from build123d import *

# Parameters (mm, degrees)
SKETCH_1_W          = 103.2
SKETCH_1_H          = 55.2
SKETCH_1_R          = 1.6
EXTRUDE_1_DEPTH     = 3
FILLET_1_R          = 2
SKETCH_2_W          = 10
SKETCH_2_H          = 8
EXTRUDE_2_DEPTH     = 10
SKETCH_3_W          = 10
SKETCH_3_H          = 7.8
SKETCH_3_W_2        = 7.907318886
SKETCH_3_H_2        = 12.798311125
SKETCH_3_W_3        = 8.73556964
SKETCH_3_H_3        = 16.298311125
SKETCH_3_H_4        = 8.73556964
EXTRUDE_3_DEPTH     = 3
SKETCH_4_R          = 2.5
SKETCH_4_W          = 7
SKETCH_4_H          = 14
SKETCH_4_W_2        = 5
SKETCH_4_H_2        = 12
EXTRUDE_4_DEPTH     = 8
SKETCH_5_R          = 0.25
EXTRUDE_5_DEPTH     = 7
SKETCH_6_R          = 5
EXTRUDE_6_DEPTH     = 12
SKETCH_7_W          = 36.530578683
SKETCH_7_H          = 32.729234011
CUT_EXTRUDE_1_DEPTH = 60.73541663


with BuildPart() as part:
    # 草图1 → 凸台-拉伸1 (new body)
    with BuildSketch(Plane(origin=(0, 0, 0), x_dir=(1, 0, 0), z_dir=(0, 1, 0))):
        Rectangle(SKETCH_1_W, SKETCH_1_H)
        with Locations(Location((-46.6, 21.6, 0), (0, 0, 270))):
            Circle(SKETCH_1_R, mode=Mode.SUBTRACT)
        with Locations(Location((46.6, 21.6, 0), (0, 0, 270))):
            Circle(SKETCH_1_R, mode=Mode.SUBTRACT)
        with Locations(Location((46.6, -21.6, 0), (0, 0, 270))):
            Circle(SKETCH_1_R, mode=Mode.SUBTRACT)
        with Locations(Location((-46.6, -21.6, 0), (0, 0, 270))):
            Circle(SKETCH_1_R, mode=Mode.SUBTRACT)
    extrude(amount=EXTRUDE_1_DEPTH)

    # 圆角1
    fillet_1_edges = [part.edges().sort_by_distance(p)[0] for p in [
        (51.6, 1.5, 27.6),
        (-51.6, 1.5, 27.6),
        (-51.6, 1.5, -27.6),
        (51.6, 1.5, -27.6),
    ]]
    fillet(fillet_1_edges, radius=FILLET_1_R)

    # 草图2 → 凸台-拉伸2 (add)
    with BuildSketch(Plane(origin=(0, 3, 0), x_dir=(1, 0, 0), z_dir=(0, 1, 0))):
        with Locations((-45.6, 13)):
            Rectangle(SKETCH_2_W, SKETCH_2_H)
        with Locations((45.6, 13)):
            Rectangle(SKETCH_2_W, SKETCH_2_H)
        with Locations((45.6, -13)):
            Rectangle(SKETCH_2_W, SKETCH_2_H)
        with Locations((-45.6, -13)):
            Rectangle(SKETCH_2_W, SKETCH_2_H)
    extrude(amount=EXTRUDE_2_DEPTH)

    # 草图3 → 凸台-拉伸3 (add)
    with BuildSketch(Plane(origin=(0, 3, 0), x_dir=(1, 0, 0), z_dir=(0, 1, 0))):
        with Locations((31, 21)):
            Rectangle(SKETCH_3_W, SKETCH_3_H)
        with Locations((-31, 21)):
            Rectangle(SKETCH_3_W, SKETCH_3_H)
        with Locations((31, 7)):
            Rectangle(SKETCH_3_W, SKETCH_3_H)
        with Locations((31, -7)):
            Rectangle(SKETCH_3_W, SKETCH_3_H)
        with Locations((31, -21)):
            Rectangle(SKETCH_3_W, SKETCH_3_H)
        with Locations((-31, 7)):
            Rectangle(SKETCH_3_W, SKETCH_3_H)
        with Locations((-31, -7)):
            Rectangle(SKETCH_3_W, SKETCH_3_H)
        with Locations((-31, -21)):
            Rectangle(SKETCH_3_W, SKETCH_3_H)
        with Locations((7.453659443, -2.077902605)):
            Rectangle(SKETCH_3_W_2, SKETCH_3_H_2)
        with Locations((-7.86778482, -3.827902605)):
            Rectangle(SKETCH_3_W_3, SKETCH_3_H_3)
        with Locations((-7.86778482, -20.98502184)):
            Rectangle(SKETCH_3_W_3, SKETCH_3_H_4)
    extrude(amount=EXTRUDE_3_DEPTH)

    # 草图4 → 凸台-拉伸4 (add)
    # profile 1 of 3: a face of its own
    with BuildSketch(Plane(origin=(0, 3, 0), x_dir=(1, 0, 0), z_dir=(0, 1, 0))):
        with Locations(Location((2, -24, 0), (0, 0, 90))):
            Circle(SKETCH_4_R)
    # profile 2 of 3: a face of its own
    with BuildSketch(Plane(origin=(0, 3, 0), x_dir=(1, 0, 0), z_dir=(0, 1, 0))):
        with Locations((-7, 17.9)):
            Rectangle(SKETCH_4_W, SKETCH_4_H)
        with Locations((-7, 17.9)):
            Rectangle(SKETCH_4_W_2, SKETCH_4_H_2, mode=Mode.SUBTRACT)
    # profile 3 of 3: a face of its own
    with BuildSketch(Plane(origin=(0, 3, 0), x_dir=(1, 0, 0), z_dir=(0, 1, 0))):
        with Locations((7, 17.9)):
            Rectangle(SKETCH_4_W, SKETCH_4_H)
        with Locations((7, 17.9)):
            Rectangle(SKETCH_4_W_2, SKETCH_4_H_2, mode=Mode.SUBTRACT)
    extrude(amount=EXTRUDE_4_DEPTH)

    # 草图5 → 凸台-拉伸5 (add)
    with BuildSketch(Plane(origin=(0, 3, 0), x_dir=(1, 0, 0), z_dir=(0, 1, 0))):
        with Locations(Location((-8.182313365, 22.9, 0), (0, 0, 90))):
            Circle(SKETCH_5_R)
        with Locations(Location((-5.817686635, 22.9, 0), (0, 0, 90))):
            Circle(SKETCH_5_R)
        with Locations(Location((-8.182313365, 20.4, 0), (0, 0, 90))):
            Circle(SKETCH_5_R)
        with Locations(Location((-5.817686635, 20.4, 0), (0, 0, 90))):
            Circle(SKETCH_5_R)
        with Locations(Location((-8.182313365, 17.9, 0), (0, 0, 90))):
            Circle(SKETCH_5_R)
        with Locations(Location((-5.817686635, 17.9, 0), (0, 0, 90))):
            Circle(SKETCH_5_R)
        with Locations(Location((-8.182313365, 15.4, 0), (0, 0, 90))):
            Circle(SKETCH_5_R)
        with Locations(Location((-5.817686635, 15.4, 0), (0, 0, 90))):
            Circle(SKETCH_5_R)
        with Locations(Location((-8.182313365, 12.9, 0), (0, 0, 90))):
            Circle(SKETCH_5_R)
        with Locations(Location((-5.817686635, 12.9, 0), (0, 0, 90))):
            Circle(SKETCH_5_R)
        with Locations(Location((5.817686635, 12.9, 0), (0, 0, 90))):
            Circle(SKETCH_5_R)
        with Locations(Location((8.182313365, 12.9, 0), (0, 0, 90))):
            Circle(SKETCH_5_R)
        with Locations(Location((5.817686635, 15.4, 0), (0, 0, 90))):
            Circle(SKETCH_5_R)
        with Locations(Location((8.182313365, 15.4, 0), (0, 0, 90))):
            Circle(SKETCH_5_R)
        with Locations(Location((5.817686635, 17.9, 0), (0, 0, 90))):
            Circle(SKETCH_5_R)
        with Locations(Location((8.182313365, 17.9, 0), (0, 0, 90))):
            Circle(SKETCH_5_R)
        with Locations(Location((5.817686635, 20.4, 0), (0, 0, 90))):
            Circle(SKETCH_5_R)
        with Locations(Location((8.182313365, 20.4, 0), (0, 0, 90))):
            Circle(SKETCH_5_R)
        with Locations(Location((8.182313365, 22.9, 0), (0, 0, 90))):
            Circle(SKETCH_5_R)
        with Locations(Location((5.817686635, 22.9, 0), (0, 0, 90))):
            Circle(SKETCH_5_R)
    extrude(amount=EXTRUDE_5_DEPTH)

    # 草图6 → 凸台-拉伸6 (add)
    with BuildSketch(Plane(origin=(0, 3, 0), x_dir=(1, 0, 0), z_dir=(0, 1, 0))):
        with Locations(Location((8.346758727, -16.964516113, 0), (0, 0, 90))):
            Circle(SKETCH_6_R)
    extrude(amount=EXTRUDE_6_DEPTH)

    # 草图7 → 切除-拉伸1 (cut, through all)
    with BuildSketch(Plane(origin=(0, 3, 0), x_dir=(1, 0, 0), z_dir=(0, 1, 0))):
        with Locations((40.691092522, -17.246006906)):
            Rectangle(SKETCH_7_W, SKETCH_7_H)
    extrude(amount=CUT_EXTRUDE_1_DEPTH, mode=Mode.SUBTRACT)


solid = part.part
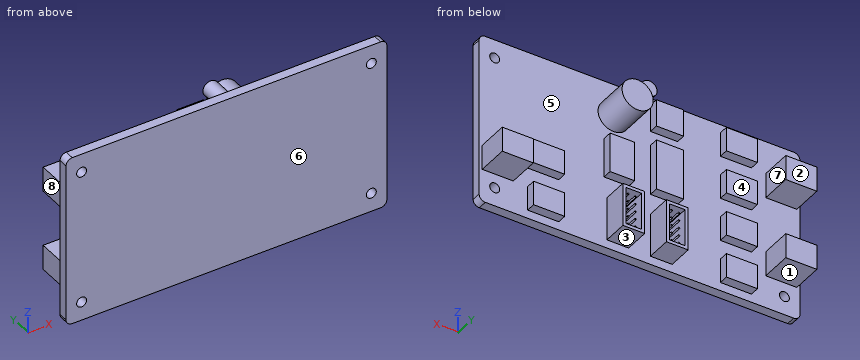
Model file for the job. Use its own axes, mm. Face numbers are marked on the shaded views. A direction names the side the tool comes from. Coordinates: 2 decimals unless noted, no trailing zeros. Write each loop counter-clockwise with the first axis right and the second up, starting at its lowest first coordinate (ties: lowest second). Pieces come first, ordered by that corner, then holes. Notation, with made-up numbers: (67, 47.25) -> (74, 47.25) arc R15 cw to (74, 70.25) -> close; hole circle Ø2 at (44.25, 10). An arc over 180 degrees is marked (long way). One line per item, written item: value. Start each with the question number.
1) Which spindle directions (+Z, -Z, +X, -X, +Y, -Y) get a long thin tool onto all of the face, cutting with end or side? Do the marked faces 1, 2, 3 and 4. Say none if no direction does.
2) Flat gauge pins, fed straight in: pin 1 Ø1.5 at (x, y) = (-33.5, 4.5) entering from +Z; pin 2 Ø3 at (x, y) = (10.5, 6) entering from +Z; pin 3 Ø6.5 at (y, z) = (8, -18.5) entering from +X. Where does each tip first touch, or does it go through?
3) Slice it at B-B on x = 2. Write the cut outline in (y, z), then the cut area to 3 significant figures.
4) Probe probe 1 along X at (y, z) = (0.85, 21.6); probe 2 along X at (y, z) = (4, 24); probe 3 along X at (y, z) = (9, -12). List the from-to ranges inside material, lowest first.
5) Pull direction X, two halves, no side cores. Call the marked faces 5, 6, 7 and 8: +X half, -X half, draft (parallel to the pull), parting line (faces both ways), or undercut.
6) Slice it at A-A on x = -46.6. Write the cut outline in (y, z).
7) Slice it at D-D on x = -27. Write the cut outline in (y, z), then the cut area to 3 significant figures.
8) Slice it at C-C on x = 46.6. Write the cut outline in (y, z).
Answers follow:
1. face 1: -Z, -X, +Y
1. face 2: +Z, -Z, -X, +Y
1. face 3: -Z, +X, -X, +Y
1. face 4: +Z, -Z, +X, +Y
2. pin 1: z = 24.9
2. pin 2: z = 21.92
2. pin 3: x = 50.6
3. outline: (0, -27.6) -> (3, -27.6) -> (3, 21.5) -> (11, 21.5) -> (11, 26.5) -> (3, 26.5) -> (3, 27.6) -> (0, 27.6) -> close
3. area: 206 mm2
4. probe 1: -51.6 to -48.2, -45 to 45, 48.2 to 51.6
4. probe 2: -36 to -26, -12.24 to -3.5, -0.5 to 4.5
4. probe 3: -50.6 to -40.6, -10.5 to -9.5, -4.5 to -3.5, 3.5 to 4.5, 9.5 to 10.5, 40.6 to 50.6
5. face 5: undercut
5. face 6: draft
5. face 7: undercut
5. face 8: -X half
6. outline: (0, -27.6) -> (3, -27.6) -> (3, -23.2) -> (0, -23.2) -> close; (0, -20) -> (3, -20) -> (3, -17) -> (13, -17) -> (13, -9) -> (3, -9) -> (3, 9) -> (13, 9) -> (13, 17) -> (3, 17) -> (3, 20) -> (0, 20) -> close; (0, 23.2) -> (3, 23.2) -> (3, 27.6) -> (0, 27.6) -> close
7. outline: (0, -27.6) -> (3, -27.6) -> (3, -24.9) -> (6, -24.9) -> (6, -17.1) -> (3, -17.1) -> (3, -10.9) -> (6, -10.9) -> (6, -3.1) -> (3, -3.1) -> (3, 3.1) -> (6, 3.1) -> (6, 10.9) -> (3, 10.9) -> (3, 17.1) -> (6, 17.1) -> (6, 24.9) -> (3, 24.9) -> (3, 27.6) -> (0, 27.6) -> close
7. area: 259 mm2
8. outline: (0, -27.6) -> (3, -27.6) -> (3, -23.2) -> (0, -23.2) -> close; (0, -20) -> (3, -20) -> (3, -17) -> (13, -17) -> (13, -9) -> (3, -9) -> (3, 20) -> (0, 20) -> close; (0, 23.2) -> (3, 23.2) -> (3, 27.6) -> (0, 27.6) -> close
